Design review of the part built by this model. Coordinates are the model's own, in mm. Round coordinates to 2 decimals unless told otherwise and drop trailing zeros. Loops run counter-clockwise (first coordinate to the right, second up) from the corner with the lowest first, then second, coordinate; pieces in that order, holes last. Notation, with made-up numbers: (35, 87.25) - (72, 87.25) arc R26 ccw to (72, 115.25) - close; hole circle Ø4 at (81, 8). An arc over 180 degrees is marked (long way). Return JSON: item names as keys, results as strings. Group by question number.
from build123d import *

# Parameters (mm, degrees)
SKETCH2_R           = 3.175
BOSS_EXTRUDE1_DEPTH = 6.35
FILLET1_R           = 5


with BuildPart() as part:
    # Sketch2 → Boss-Extrude1 (new body)
    with BuildSketch(Plane(origin=(0, 0, 0), x_dir=(0, 0, -1), z_dir=(1, 0, 0))):
        with BuildLine():
            Line((-58.176437282, 10), (-12.776437282, 10))
            ThreePointArc((-12.776437282, 10), (-2.776437282, 0), (-12.776437282, -10))
            Line((-12.776437282, -10), (-58.176437282, -10))
            ThreePointArc((-58.176437282, -10), (-68.176437282, 0), (-58.176437282, 10))
        make_face()
        with Locations((-32.776437282, 0)):
            Circle(SKETCH2_R, mode=Mode.SUBTRACT)
        with Locations((-12.776437282, 0)):
            Circle(SKETCH2_R, mode=Mode.SUBTRACT)
        with Locations((-58.176437282, 0)):
            Circle(SKETCH2_R, mode=Mode.SUBTRACT)
    extrude(amount=BOSS_EXTRUDE1_DEPTH)

    # Fillet1
    fillet1_edges = [part.edges().sort_by_distance(p)[0] for p in [
        (0, 10, 35.476437282),
        (0, 0, 2.776437282),
        (0, -10, 35.476437282),
        (0, 0, 68.176437282),
    ]]
    fillet(fillet1_edges, radius=FILLET1_R)


solid = part.part
Q1. Add section A-A, the plane z = 35. State the section outline as (x, y) points, plus the area to 3 significant figures.
Q2. Insertion check: pin 1 Ø3 at (x, y) = (3, -3.5) entering from +Z; pin 2 Ø1 at (x, y) = (5, -8) entering from +Z; pin 3 Ø5 at (y, z) = (-0.5, 17.5) entering from -X; pin 4 Ø1.5 at (x, z) = (2, 10) entering from +Y. Each pin has a flat end and moves straight along its axis. Give the tip position at first contact, or say it passes through.
Q3. Add section B-B, the plane y = 0. Give the number of separate pieces and of enclosed holes in the cut face, plus the area to 3 significant figures.
Q4. Draft analysis for pull direction Z (two halves, no side actions). For faces 1 (the cylindrical face through (5.666, -0.22, 68.174)), 2 (the cylindrical face through (3.131, -1.216, 29.844)), 3 (the flat face through (6, -10, 35)), 4 (the cylindrical face through (5.67, 0.22, 2.78)), state which applies: pulls with the +Z half, pulls with the -Z half, needs draft (parallel to the pull), parting line crosses it, or undercut.
Q5. For line 1 (Z direction, x = 1.5, y = -0.25); line 2 (Z direction, x = 5, y = -0.75); line 3 (X direction, y = 5.25, z = 21), list the stretches that pass through material, from the lowest coordinate up.
Evaluation:
{
 "1": {"outline": "(0, -5) arc R5 ccw to (5, -10) - (6.35, -10) - (6.35, -2.27) - (0, -2.27) - close; (0, 2.27) - (6.35, 2.27) - (6.35, 10) - (5, 10) arc R5 ccw to (0, 5) - close", "area": "87.5 mm²"},
 "2": {"pin 1": "z = 67.78", "pin 2": "z = 64.79", "pin 3": "x = 0", "pin 4": "y = 9.1"},
 "3": {"separate pieces": "4", "enclosed holes": "0", "area": "284 mm²"},
 "4": {"face 1": "pulls with the +Z half", "face 2": "undercut", "face 3": "needs draft", "face 4": "pulls with the -Z half"},
 "5": {"line 1": "4.21 to 9.61, 15.94 to 29.61, 35.94 to 55.01, 61.34 to 66.74", "line 2": "2.8 to 9.69, 15.86 to 29.69, 35.86 to 55.09, 61.26 to 68.15", "line 3": "0.01 to 6.35"}
}
